Verification items for the finished model (mm, model axes). Face numbers are marked on the shaded views. A direction names the side the tool comes from. Round coordinates to 2 decimals unless told otherwise and drop trailing zeros. Order: outer loops, then holes, each group sorted by start corner. A loop starts at its lowest first (then second) coordinate and runs counter-clockwise, first axis right, second up. Notation, with made-up numbers: (57.5, -23.5) -> (81.5, -23.5) arc R9 cw to (81.5, -7.5) -> close; hole circle Ø10 at (11.25, 52). An arc over 180 degrees is marked (long way). Return JSON: item names as keys, results as strings. Group by question number.
1) Draft check along X on the marked faces 1, 2, 3 and 4. Enter one of: pulls with the +X half, pulls with the -X half, needs draft (parallel to the pull), parting line crosses it, or undercut.
2) Tool access check on the marked faces 5 and 6. Record the directions out of +Z, -Z, +X, -X, +Y, -Y that give a thin tool (end or side, any length) a straight path to the whole face; none if there is none.
3) Section check A-A on z = -9. Enter the section's corners in (x, y).
4) Section check C-C on z = -33. Enter the section's corners in (x, y).
5) Depth check by flat-ended pin: pin 1 (3 mm diameter, centred on y = 7, z = -38.5, fed in from -X); pin 2 (3 mm diameter, centred on y = 6, z = 27, fed in from -X); pin 3 (5 mm diameter, centred on x = -26.5, z = -17.5, fed in from -Y); pin 4 (5 mm diameter, centred on y = 4.5, z = -17, fed in from +X). Enter the tip coordinate at first touch or a pass-through.
6) Scan lines: L1, parallel to Z at x = 17.5, y = 6.25; L2, parallel to Z at x = -37, y = 1.5; L3, parallel to X at y = 6.25, z = -3. Record each from-to range of solid material in increasing order.
7) Section check B-B on y = 7.5. State how many separate pieces and enclosed holes the cut face has, plus the area to 3 significant figures.
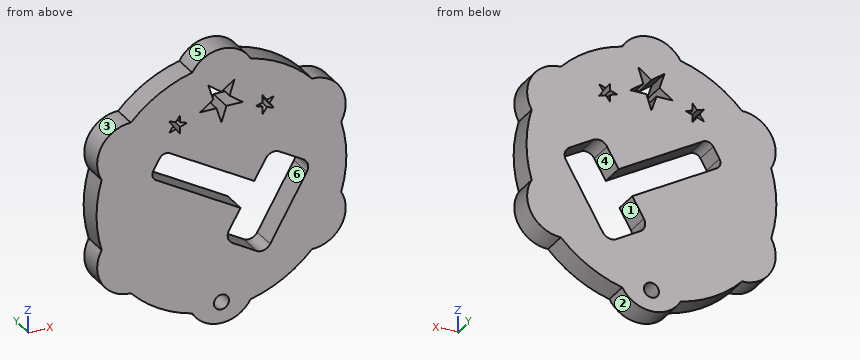
```python
from build123d import *

# Parameters (mm, degrees)
SKETCH1_R           = 3
BOSS_EXTRUDE1_DEPTH = 10


with BuildPart() as part:
    # Sketch1 → Boss-Extrude1 (new body)
    with BuildSketch(Plane(origin=(0, 0, 0), x_dir=(1, 0, 0), z_dir=(0, 1, 0))):
        with BuildLine():
            ThreePointArc((-11.691342951, 48.613912618), (-25, 43.301270189), (-36.255211829, 34.431956309))
            ThreePointArc((-36.255211829, 34.431956309), (-47.94655478, 27.681956309), (-47.94655478, 14.181956309))
            ThreePointArc((-47.94655478, 14.181956309), (-50, 0), (-47.94655478, -14.181956309))
            ThreePointArc((-47.94655478, -14.181956309), (-47.94655478, -27.681956309), (-36.255211829, -34.431956309))
            ThreePointArc((-36.255211829, -34.431956309), (-25, -43.301270189), (-11.691342951, -48.613912618))
            ThreePointArc((-11.691342951, -48.613912618), (0, -55.363912618), (11.691342951, -48.613912618))
            ThreePointArc((11.691342951, -48.613912618), (25, -43.301270189), (36.255211829, -34.431956309))
            ThreePointArc((36.255211829, -34.431956309), (47.94655478, -27.681956309), (47.94655478, -14.181956309))
            ThreePointArc((47.94655478, -14.181956309), (50, 0), (47.94655478, 14.181956309))
            ThreePointArc((47.94655478, 14.181956309), (47.94655478, 27.681956309), (36.255211829, 34.431956309))
            ThreePointArc((36.255211829, 34.431956309), (25, 43.301270189), (11.691342951, 48.613912618))
            ThreePointArc((11.691342951, 48.613912618), (0, 55.363912618), (-11.691342951, 48.613912618))
        make_face()
        with Locations(Location((0, 46.863912618, 0), (0, 0, 270))):
            Circle(SKETCH1_R, mode=Mode.SUBTRACT)
        with BuildLine():
            Line((-27.230762114, -12.834936491), (-24.730762114, -17.165063509))
            ThreePointArc((-24.730762114, -17.165063509), (-22.909143037, -18.562840988), (-20.632685902, -18.263139721))
            Line((-20.632685902, -18.263139721), (13.142304845, 1.236860279))
            Line((13.142304845, 1.236860279), (17.742304845, -6.730573436))
            ThreePointArc((17.742304845, -6.730573436), (20.17113028, -8.594276741), (23.206406461, -8.194675051))
            Line((23.206406461, -8.194675051), (32.732685902, -2.694675051))
            ThreePointArc((32.732685902, -2.694675051), (34.596389207, -0.265849616), (34.196787517, 2.769426564))
            Line((34.196787517, 2.769426564), (19.496787517, 28.230573436))
            ThreePointArc((19.496787517, 28.230573436), (17.067962083, 30.094276741), (14.032685902, 29.694675051))
            Line((14.032685902, 29.694675051), (4.506406461, 24.194675051))
            ThreePointArc((4.506406461, 24.194675051), (2.642703155, 21.765849616), (3.042304845, 18.730573436))
            Line((3.042304845, 18.730573436), (7.642304845, 10.763139721))
            Line((7.642304845, 10.763139721), (-26.132685902, -8.736860279))
            ThreePointArc((-26.132685902, -8.736860279), (-27.530463381, -10.558479355), (-27.230762114, -12.834936491))
        make_face(mode=Mode.SUBTRACT)
        Polygon((-2.008610463, -31.818132644), (0, -25.636265288), (2.008610463, -31.818132644), (8.508610463, -31.818132644), (3.25, -35.638736784), (5.258610463, -41.82060414), (0, -38), (-5.258610463, -41.82060414), (-3.25, -35.638736784), (-8.508610463, -31.818132644), align=None, mode=Mode.SUBTRACT)
        Polygon((13.742304845, -28.81792347), (16.506236868, -27.919867517), (16.506236868, -25.013697405), (18.2144408, -27.364838414), (20.978372823, -26.466782461), (19.27016889, -28.81792347), (20.978372823, -31.16906448), (18.2144408, -30.271008526), (16.506236868, -32.622149536), (16.506236868, -29.715979424), align=None, mode=Mode.SUBTRACT)
        Polygon((-13.742304845, -28.81792347), (-16.506236868, -27.919867517), (-16.506236868, -25.013697405), (-18.2144408, -27.364838414), (-20.978372823, -26.466782461), (-19.27016889, -28.81792347), (-20.978372823, -31.16906448), (-18.2144408, -30.271008526), (-16.506236868, -32.622149536), (-16.506236868, -29.715979424), align=None, mode=Mode.SUBTRACT)
    extrude(amount=BOSS_EXTRUDE1_DEPTH)


solid = part.part
```
Check result:
{
 "1": {"face 1": "undercut", "face 2": "parting line crosses it", "face 3": "pulls with the -X half", "face 4": "undercut"},
 "2": {"face 5": "+Z, +Y, -Y", "face 6": "+Y, -Y"},
 "3": {"outline": "(-49.18, 0) -> (4.59, 0) -> (4.59, 10) -> (-49.18, 10) -> close; (30.6, 0) -> (49.18, 0) -> (49.18, 10) -> (30.6, 10) -> close"},
 "4": {"outline": "(-42.31, 0) -> (42.31, 0) -> (42.31, 10) -> (-42.31, 10) -> close"},
 "5": {"pin 1": "x = -33.63", "pin 2": "x = -48.96", "pin 3": "y = 0", "pin 4": "x = 49.68"},
 "6": {"L1": "-46.84 to -29.95, 6.31 to 26.38, 31.25 to 46.84", "L2": "-34.41 to 34.41", "L3": "-49.91 to -5.8, 34.06 to 49.91"},
 "7": {"separate pieces": "1", "enclosed holes": "5", "area": "7,090 mm^2"}
}
